```python
from build123d import *

# Parameters (mm, degrees)
SKETCH1_R           = 4.3307
BOSS_EXTRUDE1_DEPTH = 0.79375
SKETCH2_R           = 0.93345
BOSS_EXTRUDE2_DEPTH = 4.7625


with BuildPart() as part:
    # Sketch1 → Boss-Extrude1 (new body)
    with BuildSketch(Plane(origin=(0, 0, 0), x_dir=(1, 0, 0), z_dir=(0, 1, 0))):
        with BuildLine():
            Line((-1.7272, -14.3256), (1.7272, -14.3256))
            Line((1.7272, -14.3256), (1.7272, -8.578734844))
            ThreePointArc((1.7272, -8.578734844), (2.225592247, -6.457699407), (3.616456198, -4.780593679))
            ThreePointArc((3.616456198, -4.780593679), (0, 5.9944), (-3.616456198, -4.780593679))
            ThreePointArc((-3.616456198, -4.780593679), (-2.225592247, -6.457699407), (-1.7272, -8.578734844))
            Line((-1.7272, -8.578734844), (-1.7272, -14.3256))
        make_face()
        Circle(SKETCH1_R, mode=Mode.SUBTRACT)
    extrude(amount=BOSS_EXTRUDE1_DEPTH)

    # Sketch2 → Boss-Extrude2 (add)
    with BuildSketch(Plane.XY.offset(14.3256)):
        with BuildLine():
            Line((-1.7272, 0), (-1.7272, 1.7272))
            ThreePointArc((-1.7272, 1.7272), (0, 3.4544), (1.7272, 1.7272))
            Line((1.7272, 1.7272), (1.7272, 0))
            Line((1.7272, 0), (-1.7272, 0))
        make_face()
        with Locations((0, 1.7272)):
            Circle(SKETCH2_R, mode=Mode.SUBTRACT)
    extrude(amount=-BOSS_EXTRUDE2_DEPTH)


solid = part.part
```
The model under review builds one solid part; all positions refer to its coordinate system, in mm. A direction names the side the tool comes from. Round coordinates to 2 decimals unless told otherwise and drop trailing zeros. Loops run counter-clockwise (first coordinate to the right, second up) from the corner with the lowest first, then second, coordinate; pieces in that order, holes last.
1) Consider section A-A on z = 0. State the section outline as (x, y) points.
Values follow:
outline: (-5.99, 0) - (-4.33, 0) - (-4.33, 0.79) - (-5.99, 0.79) - close; (4.33, 0) - (5.99, 0) - (5.99, 0.79) - (4.33, 0.79) - close
2) Consider section C-C on y = 0.3. State the section outline as (x, z) points (1 decimal), then the cut area to 3 significant figures.
Values follow:
outline: (-3.6, 4.8) arc R6 ccw (long way) to (3.6, 4.8) arc R4.8 cw to (1.7, 8.6) - (1.7, 14.3) - (-1.7, 14.3) - (-1.7, 8.6) arc R4.8 cw to start; hole circle Ø8.7 at (0, 0)
area: 85.3 mm2
3) Consider section D-D on x = 4.75. State the section outline as (y, z) points, then the cut area to 3 significant figures.
Values follow:
outline: (0, -3.66) - (0.79, -3.66) - (0.79, 3.66) - (0, 3.66) - close
area: 5.80 mm2
4) The part is to be moulded in two halves that separate along Y. For faces 1 (the face through (0, 0, 5)), 2 (the face through (-0.122, 2.653, 11.978)), 3 (the face through (2.21, 0.39, 6.49)), say which applies: pulls with the +Y half, pulls with the -Y half, needs draft (parallel to the pull), parting line crosses it, or undercut.
Values follow:
face 1: pulls with the -Y half
face 2: undercut
face 3: needs draft
5) Tool access review of faces 4 (the face through (0.21, 0.39, -5.99)), 5 (the face through (0, 0.794, 5)), 6 (the face through (1.727, 1, 11)), 7 (the face through (-1.727, 1, 11)), 8 (the face through (-0.038, 3.454, 11.978)): name each direction out of +Z, -Z, +X, -X, +Y, -Y from which nothing blocks a thin tool from reaching the whole face with its end or side.
Values follow:
face 4: +Y, -Y
face 5: -Z, +X, -X, +Y
face 6: +Z, +X, +Y, -Y
face 7: +Z, -X, +Y, -Y
face 8: +Z, -Z, +Y
6) Clearance check with flat-ended pins moving along their axes: P1, Ø1.5, axis at y = 1, z = 7, coming from the +X side; P2, Ø0.9, axis at y = 1.5, z = 12.5, coming from the +X side; P3, Ø5, axis at x = 4.5, z = -2, coming from the +Y side; P4, Ø5, axis at x = 3.5, z = 6, coming from the -Y side. State where each tip first meets the part, or that it passes through.
Values follow:
P1: stops at x = 2.32
P2: stops at x = 1.73
P3: stops at y = 0.79
P4: stops at y = 0
7) Consider section B-B on y = 2.4. State the section outline as (x, z) points, then the cut area to 3 significant figures.
Values follow:
outline: (-1.59, 9.56) - (-0.65, 9.56) - (-0.65, 14.33) - (-1.59, 14.33) - close; (0.65, 9.56) - (1.59, 9.56) - (1.59, 14.33) - (0.65, 14.33) - close
area: 8.99 mm2
8) Wall thickness on line 1 along Y through (x, z) = (0, 12); line 2 along Z through (x, y) = (0, 0.2); line 3 along X through (y, z) = (0.2, 0): over which ranges is each line inside the solid? List them lowest first.
Values follow:
line 1: y = 0 to 0.79, 2.66 to 3.45
line 2: z = -5.99 to -4.33, 4.33 to 14.33
line 3: x = -5.99 to -4.33, 4.33 to 5.99
